Could you check a few things on this model? Use its own coordinates, in mm. Face numbers are marked on the shaded views. A direction names the side the tool comes from. Give positions to 0.01 mm unless a question says otherwise; leave off trailing zeros. Loops run counter-clockwise (first coordinate to the right, second up) from the corner with the lowest first, then second, coordinate; pieces in that order, holes last. Notation, with made-up numbers: M 76,-3 L 99,-3 A10 cw 99,13 Z; hole C 73,67 d5. An arc over 180 degrees is marked long. Use a Markdown table: item, result. Add a question column.
1) Suppose I cut it at C-C on x = -231. List the corners of the cut face in (y, z) for me.
2) Will these pins go through, and if not, where does the flat tip stop? pin 1 Ø19 at (x, y) = (20, 14.5) entering from +Z; pin 2 Ø1.5 at (y, z) = (20, -42) entering from +X; pin 3 Ø3 at (x, y) = (-125.41, -31.75) entering from +Z; pin 4 Ø8 at (y, z) = (-34, -54.5) entering from -X.
3) We'd pull the mould along X, two halves only. Please class the marked faces 4, 5 and 6: +X half, -X half, draft (parallel to the pull), parting line (faces both ways), or undercut.
4) Which directions (+Z, -Z, +X, -X, +Y, -Y) give clear straight access to the entire face, cutting with the end or side of a thin tool? Please do the marked faces 1, 2 and 3.
5) Suppose I cut it at A-A on y = -19.05. Count the separate pieces of the cut face and the enclosed holes in it, and give its area (3 significant figures).
6) If I drill on line 1 along X through (y, z) = (8.5, -35) (1 decimal); line 2 along Z through (x, y) = (-188, 35.5); line 3 along X through (y, z) = (-19, -72), over which ranges is the centre line in solid material (lowest first)? Write a range as [from, to].
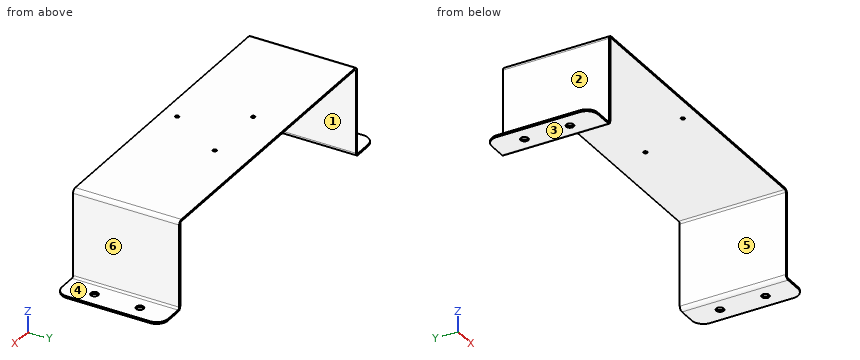
```python
from build123d import *

# Parameters (mm, degrees)
F1_DEPTH = 44.45
F2_R     = 3.175
F2_R_2   = 1.5875
F3_DEPTH = 75.40725
F4_R     = 9.525


with BuildPart() as f1:
    # F0 (on Front) → F1 (new body, symmetric)
    with BuildSketch(Plane.XZ):
        with BuildLine():
            Line((-125.4125, 0), (-1.5875, 0))
            ThreePointArc((-1.5875, 0), (-0.4649679849, -0.4649679849), (0, -1.5875))
            Line((0, -1.5875), (0, -70.64375))
            ThreePointArc((0, -70.64375), (0.9299359697, -72.8888140303), (3.175, -73.81875))
            Line((3.175, -73.81875), (26.9875, -73.81875))
            Line((26.9875, -73.81875), (26.9875, -72.23125))
            Line((26.9875, -72.23125), (3.175, -72.23125))
            ThreePointArc((3.175, -72.23125), (2.0524679849, -71.7662820151), (1.5875, -70.64375))
            Line((1.5875, -70.64375), (1.5875, -1.5875))
            ThreePointArc((1.5875, -1.5875), (0.6575640303, 0.6575640303), (-1.5875, 1.5875))
            Line((-1.5875, 1.5875), (-125.4125, 1.5875))
            Line((-125.4125, 1.5875), (-249.2375, 1.5875))
            ThreePointArc((-249.2375, 1.5875), (-251.4825640303, 0.6575640303), (-252.4125, -1.5875))
            Line((-252.4125, -1.5875), (-252.4125, -70.64375))
            ThreePointArc((-252.4125, -70.64375), (-252.8774679849, -71.7662820151), (-254, -72.23125))
            Line((-254, -72.23125), (-277.8125, -72.23125))
            Line((-277.8125, -72.23125), (-277.8125, -73.81875))
            Line((-277.8125, -73.81875), (-254, -73.81875))
            ThreePointArc((-254, -73.81875), (-251.7549359697, -72.8888140303), (-250.825, -70.64375))
            Line((-250.825, -70.64375), (-250.825, -1.5875))
            ThreePointArc((-250.825, -1.5875), (-250.3600320151, -0.4649679849), (-249.2375, 0))
            Line((-249.2375, 0), (-125.4125, 0))
        make_face()
    extrude(amount=F1_DEPTH, both=True)

    # F2 (on face) → F3 (cut, through all)
    with BuildSketch(Plane.XY.offset(1.5875)):
        with Locations((14.2875, 19.05)):
            Circle(F2_R)
        with Locations((14.2875, -19.05)):
            Circle(F2_R)
        with Locations((-125.4125, -31.75)):
            Circle(F2_R_2)
        with Locations((-97.9161934298, 15.875)):
            Circle(F2_R_2)
        with Locations((-152.9088065702, 15.875)):
            Circle(F2_R_2)
        with Locations((-265.1125, 19.05)):
            Circle(F2_R)
        with Locations((-265.1125, -19.05)):
            Circle(F2_R)
    extrude(amount=-F3_DEPTH, mode=Mode.SUBTRACT)

    # F4
    f4_edges = [f1.edges().sort_by_distance(p)[0] for p in [
        (26.9875, 44.45, -73.025),
        (26.9875, -44.45, -73.025),
        (-277.8125, -44.45, -73.025),
        (-277.8125, 44.45, -73.025),
    ]]
    fillet(f4_edges, radius=F4_R)


solid = f1.part
```
Answer block:
| question | item | result |
|---|---|---|
| 1 | outline | M -44.45,0 L 44.45,0 L 44.45,1.59 L -44.45,1.59 Z |
| 2 | pin 1 | stops at z = -72.23 |
| 2 | pin 2 | stops at x = 1.59 |
| 2 | pin 3 | passes through |
| 2 | pin 4 | stops at x = -252.41 |
| 3 | face 4 | draft |
| 3 | face 5 | undercut |
| 3 | face 6 | +X half |
| 4 | face 1 | -Z, +Y, -Y |
| 4 | face 2 | +Z, -X, +Y, -Y |
| 4 | face 3 | -Z, +X, -X, +Y, -Y |
| 5 | separate pieces | 3 |
| 5 | enclosed holes | 0 |
| 5 | area | 692 mm^2 |
| 6 | line 1 | x = [-252.4, -250.8], [0, 1.6] |
| 6 | line 2 | z = [0, 1.59] |
| 6 | line 3 | x = [-253.17, -251.13], [0.3, 2.35] |
